Part model, mm, in its own coordinate system. A direction names the side the tool comes from. Coordinates: 2 decimals unless noted, no trailing zeros. Loops run counter-clockwise (first coordinate to the right, second up) from the corner with the lowest first, then second, coordinate; pieces in that order, holes last.
```python
from build123d import *

# Parameters (mm, degrees)
SKETCH_1_W          = 170
SKETCH_1_H          = 60
SKETCH_1_R          = 1.5
EXTRUDE_1_DEPTH     = 5
SKETCH_2_R          = 2.5
CUT_EXTRUDE_1_DEPTH = 5
SKETCH_3_W          = 170
SKETCH_3_H          = 26
CUT_EXTRUDE_2_DEPTH = 10
SKETCH_4_W          = 18
SKETCH_4_H          = 12
CUT_EXTRUDE_3_DEPTH = 10
FILLET_1_R          = 3
SKETCH_5_W          = 170
SKETCH_5_H          = 4
CUT_EXTRUDE_4_DEPTH = 91.277350426
FILLET_2_R          = 8


with BuildPart() as part:
    # 草图1 → 凸台-拉伸1 (new body)
    with BuildSketch(Plane.XY):
        Rectangle(SKETCH_1_W, SKETCH_1_H)
        with Locations((-77, -8)):
            Circle(SKETCH_1_R, mode=Mode.SUBTRACT)
        with Locations((-77, -1)):
            Circle(SKETCH_1_R, mode=Mode.SUBTRACT)
        with Locations(Location((77, -1, 0), (0, 0, 180))):
            Circle(SKETCH_1_R, mode=Mode.SUBTRACT)
        with Locations(Location((77, -8, 0), (0, 0, 180))):
            Circle(SKETCH_1_R, mode=Mode.SUBTRACT)
    extrude(amount=EXTRUDE_1_DEPTH)

    # 草图2 → 切除-拉伸1 (cut)
    with BuildSketch(Plane.XY.offset(5)):
        with Locations((-30, -20)):
            Circle(SKETCH_2_R)
        with Locations((30, -20)):
            Circle(SKETCH_2_R)
    extrude(amount=-CUT_EXTRUDE_1_DEPTH, mode=Mode.SUBTRACT)

    # 草图3 → 切除-拉伸2 (cut)
    with BuildSketch(Plane.XY.offset(5)):
        with Locations((0, 17)):
            Rectangle(SKETCH_3_W, SKETCH_3_H)
    extrude(amount=-CUT_EXTRUDE_2_DEPTH, mode=Mode.SUBTRACT)

    # 草图4 → 切除-拉伸3 (cut)
    with BuildSketch(Plane.XY.offset(5)):
        with Locations((-63, -12)):
            Rectangle(SKETCH_4_W, SKETCH_4_H)
        with Locations((63, -12)):
            Rectangle(SKETCH_4_W, SKETCH_4_H)
    extrude(amount=-CUT_EXTRUDE_3_DEPTH, mode=Mode.SUBTRACT)

    # 圆角1
    fillet_1_edges = [part.edges().sort_by_distance(p)[0] for p in [
        (-72, -18, 2.5),
        (-72, -6, 2.5),
        (-54, -6, 2.5),
        (-54, -18, 2.5),
        (72, -6, 2.5),
        (72, -18, 2.5),
        (54, -18, 2.5),
        (54, -6, 2.5),
    ]]
    fillet(fillet_1_edges, radius=FILLET_1_R)

    # 草图5 → 切除-拉伸4 (cut, through all)
    with BuildSketch(Plane.XY.offset(5)):
        with Locations((0, -28)):
            Rectangle(SKETCH_5_W, SKETCH_5_H)
    extrude(amount=-CUT_EXTRUDE_4_DEPTH, mode=Mode.SUBTRACT)

    # 圆角2
    fillet_2_edges = [part.edges().sort_by_distance(p)[0] for p in [
        (-85, -26, 2.5),
        (85, -26, 2.5),
        (-85, 4, 2.5),
        (85, 4, 2.5),
    ]]
    fillet(fillet_2_edges, radius=FILLET_2_R)


solid = part.part
```
Q1. Saw through at A-A (x = 30). List the corners of the cut face in (y, z).
Q2. Tool access for faces 1 (the cylindrical face through (-71.1, -6.86, 2.46)), 2 (the flat face through (-1, 4, 3)): list every direction of +Z, -Z, +X, -X, +Y, -Y with a clear straight run to the whole face (end or side of a thin tool).
Q3. Mould opens along X. For faces 3 (the cylindrical face through (71.1, -17.14, 2.46)), 4 (the cylindrical face through (-82.719, 1.594, 2.465)), 5 (the cylindrical face through (82.594, 1.719, 2.465)) say: released by +X, released by -X, zero draft, split by the parting line, or undercut.
Q4. Probe line 1 (Y direction, x = -77, z = 1.55); line 2 (Y direction, x = -30, z = 3.5); line 3 (X direction, y = -1.5, z = 4.8). List the from-to ranges inside material, lowest first.
Q5. Saw through at D-D (x = 65.5). List the corners of the cut face in (y, z), plus the area to 3 significant figures.
Q6. Saw through at C-C (y = -1). List the corners of the cut face in (x, z), plus the area to 3 significant figures.
Q7. Saw through at B-B (z = 2.15). Count the separate pieces of the cut face and the enclosed holes in it, plus the area to 3 significant figures.
Checked values:
1. outline: (-26, 0) - (-22.5, 0) - (-22.5, 5) - (-26, 5) - close; (-17.5, 0) - (4, 0) - (4, 5) - (-17.5, 5) - close
2. face 1: +Z, -Z
2. face 2: +Z, -Z, +X, -X, +Y
3. face 3: undercut
3. face 4: released by -X
3. face 5: released by +X
4. line 1: y = -26 to -9.5, -6.5 to -2.5, 0.5 to 4
4. line 2: y = -26 to -22.5, -17.5 to 4
4. line 3: x = -84.6 to -78.41, -75.59 to 75.59, 78.41 to 84.6
5. outline: (-26, 0) - (-18, 0) - (-18, 5) - (-26, 5) - close; (-6, 0) - (4, 0) - (4, 5) - (-6, 5) - close
5. area: 90.0 mm2
6. outline: (-84.42, 0) - (-78.5, 0) - (-78.5, 5) - (-84.42, 5) - close; (-75.5, 0) - (75.5, 0) - (75.5, 5) - (-75.5, 5) - close; (78.5, 0) - (84.42, 0) - (84.42, 5) - (78.5, 5) - close
6. area: 814 mm2
7. separate pieces: 1
7. enclosed holes: 8
7. area: 4,560 mm2
